Autodesk Inventor part; units mm, degrees
ref_plane "YZ Plane" through (0, 0, 0) normal (1, 0, 0) x (0, 1, 0)
ref_plane "XZ Plane" through (0, 0, 0) normal (0, 1, 0) x (-1, 0, 0)
ref_plane "XY Plane" through (0, 0, 0) normal (0, 0, 1) x (1, 0, 0)
sketch "Sketch1" plane through (0, 0, 0) normal (0, 1, 0) x (-1, 0, 0)
  line L0 (2.2807, -2.5252) -> (-23.1193, -2.5252)
  line L1 (-23.1193, -2.5252) -> (-23.1193, 48.2748)
  line L2 (-23.1193, 48.2748) -> (2.2807, 48.2748)
  line L3 (2.2807, 48.2748) -> (2.2807, -2.5252)
  line L4 (-19.9443, 0.6498) -> (-0.8943, 0.6498)
  line L5 (-0.8943, 0.6498) -> (-0.8943, 45.0998)
  line L6 (-0.8943, 45.0998) -> (-19.9443, 45.0998)
  line L7 (-19.9443, 45.0998) -> (-19.9443, 0.6498)
  point P0 (0, 0)
  dimension "d0" = 25.4
  dimension "d1" = 50.8
  dimension "d2" = 3.175
extrude "Extrusion1" add sketch "Sketch1" along normal blind 762
sketch "Sketch3" plane through (-2.2807, 0, 48.2748) normal (0, 0, 1) x (1, 0, 0)
  line L0 (22.225, 0) -> (3.175, 0) construction
  line L1 (12.7, 0) -> (12.7, 12.7) construction
  line L2 (12.7, 12.7) -> (12.7, 38.1) construction
  line L3 (12.7, 38.1) -> (12.7, 63.5) construction
  circle A0 centre (12.7, 63.5) radius 2.5797
  circle A1 centre (12.7, 38.1) radius 2.5797
  circle A2 centre (12.7, 12.7) radius 2.5797
  line L4 (12.7, 685.8) -> (12.7, 673.1) construction
  circle A3 centre (12.7, 673.1) radius 2.5797
  line L5 (12.7, 673.1) -> (12.7, 647.7) construction
  line L6 (12.7, 647.7) -> (12.7, 622.3) construction
  circle A4 centre (12.7, 647.7) radius 2.5797
  circle A5 centre (12.7, 622.3) radius 2.5797
  point P0 (2.2807, 0)
  dimension "d19" = 12.7
  dimension "d20" = 25.4
  dimension "d21" = 25.4
  dimension "d22" = 5.1594
  dimension "d23" = 5.1594
  dimension "d24" = 5.1594
  dimension "d38" = 12.7
  dimension "d39" = 5.1594
  dimension "d40" = 25.4
  dimension "d41" = 25.4
  dimension "d42" = 5.1594
  dimension "d43" = 5.1594
extrude "Extrusion3" cut sketch "Sketch3" against normal blind 762
sketch "Sketch4" plane through (23.1193, 0, 48.2748) normal (1, 0, 0) x (0, 0, -1)
  line L0 (3.175, 762) -> (47.625, 762) construction
  line L1 (25.4, 762) -> (25.4, 736.6) construction
  point P0 (48.2748, 0)
  dimension "d44" = 25.4
sketch "Sketch5" plane through (-2.2807, 0, -2.5252) normal (-1, 0, 0) x (0, 0, 1)
  circle A0 centre (25.4, 12.7) radius 2.5797
  line L0 (50.8, 0) -> (50.8, 762)
  circle A1 centre (25.4, 38.1) radius 2.5797 construction
  line L1 (50.8, 38.1) -> (38.1, 38.1) construction
  circle A2 centre (25.4, 63.5) radius 2.5797 construction
  line L2 (50.8, 63.5) -> (38.1, 63.5) construction
  circle A3 centre (38.1, 63.5) radius 2.5797
  circle A4 centre (38.1, 38.1) radius 2.5797
  circle A5 centre (38.1, 12.7) radius 2.5797
  line L3 (38.1, 12.7) -> (50.8, 12.7) construction
  circle A6 centre (25.4, 622.3) radius 2.5797 construction
  line L4 (50.8, 622.3) -> (38.1, 622.3) construction
  circle A7 centre (25.4, 647.7) radius 2.5797 construction
  line L5 (50.8, 647.7) -> (38.1, 647.7) construction
  circle A8 centre (25.4, 673.1) radius 2.5797 construction
  line L6 (50.8, 673.1) -> (38.1, 673.1) construction
  circle A9 centre (38.1, 647.7) radius 2.5797
  circle A10 centre (38.1, 622.3) radius 2.5797
  circle A11 centre (38.1, 673.1) radius 2.5797
  point P0 (2.5252, 0)
  dimension "d46" = 12.7
  dimension "d47" = 12.7
  dimension "d48" = 5.1594
  dimension "d49" = 5.1594
  dimension "d50" = 5.1594
  dimension "d51" = 12.7
  dimension "d52" = 12.7
  dimension "d53" = 12.7
  dimension "d54" = 5.1594
  dimension "d55" = 5.1594
  dimension "d56" = 5.1594
extrude "Extrusion4" cut sketch "Sketch5" against normal blind 762 contours A3 | A4 | A5 | A9 | A10 | A11
sketch "Sketch6" plane through (-2.2807, 0, -2.5252) normal (-1, 0, 0) x (0, 0, 1)
  line L0 (47.625, 762) -> (3.175, 762) construction
  line L1 (25.4, 762) -> (25.4, 736.6) construction
  circle A0 centre (25.4, 736.6) radius 14.2875
  point P0 (2.5252, 0)
  dimension "d59" = 25.4
  dimension "d60" = 28.575
extrude "Extrusion5" cut sketch "Sketch6" against normal blind 304.8
sketch "Sketch7" plane through (-2.2807, 0, -2.5252) normal (-1, 0, 0) x (0, 0, 1)
  circle A0 centre (38.1, 12.7) radius 2.5797 construction
  line L0 (38.1, 12.7) -> (38.1, 114.3) construction
  line L1 (38.1, 12.7) -> (38.1, 190.5) construction
  line L2 (38.1, 190.5) -> (12.7, 190.5) construction
  line L3 (38.1, 114.3) -> (12.7, 114.3) construction
  circle A1 centre (38.1, 190.5) radius 2.5797
  circle A2 centre (12.7, 190.5) radius 2.5797
  circle A3 centre (38.1, 114.3) radius 2.5797
  circle A4 centre (12.7, 114.3) radius 2.5797
  point P0 (2.5252, 0)
  dimension "d63" = 101.6
  dimension "d64" = 177.8
  dimension "d65" = 25.4
  dimension "d66" = 25.4
  dimension "d67" = 5.1594
  dimension "d68" = 5.1594
  dimension "d69" = 5.1594
  dimension "d70" = 5.1594
extrude "Extrusion6" cut sketch "Sketch7" against normal blind 50.8
sketch "Sketch8" plane through (-2.2807, 0, -2.5252) normal (-1, 0, 0) x (0, 0, 1)
  line L0 (0, 0) -> (6.5024, 0) construction
  line L1 (47.625, 0) -> (3.175, 0) construction
  line L2 (6.5024, 0) -> (6.5024, 6.5024) construction
  circle A0 centre (6.5024, 6.5024) radius 3.302
  line L3 (6.5024, 6.5024) -> (6.5024, 93.4974) construction
  circle A1 centre (6.5024, 93.4974) radius 3.302
  point P0 (2.5252, 0)
  dimension "d73" = 6.5024
  dimension "d74" = 6.5024
  dimension "d75" = 6.604
  dimension "d76" = 86.995
  dimension "d77" = 6.604
extrude "Extrusion7" cut sketch "Sketch8" against normal blind 50.8
properties part number "30in 1x1 Beam"
Source: CAD feature listing. Evaluate the final solid. Frame: model axes, mm. A direction names the side the tool comes from. Give positions to 0.01 mm unless a question says otherwise; leave off trailing zeros. Write each loop counter-clockwise with the first axis right and the second up, starting at its lowest first coordinate (ties: lowest second). Pieces come first, ordered by that corner, then holes. Notation, with made-up numbers: (33.5, 42.5) - (46.5, 42.5) arc R19 ccw to (46.5, 53.5) - close; hole circle Ø8 at (-12.5, 12). An arc over 180 degrees is marked (long way). One line per item, written item: value. Start each with the question number.
Q1. Section query B-B, the plane z = 22. Return the cut outline in (x, y).
Q2. Set-up query: faces 4 (the face through (19.944, 376, 23)), 5 (the face through (21.51, 722.65, 19.78)). Return all of +Z, -Z, +X, -X, +Y, -Y with unobstructed straight access to the full face (end or side cutting, diameter ignored); none if empty.
Q3. Material intervals for probe 1 along Z at (x, y) = (-1.1, 190.5); probe 2 along Y at (x, z) = (20.5, 3.5); probe 3 along Z at (x, y) = (17.5, 506), sorted ascending. Write a range as from..to.
Q4. Section query C-C, the plane y = 268. Return the cut outline in (x, z), then the cut area to 3 significant figures.
Q5. First-contact query: pin 1 Ø8.5 at (x, y) = (10.42, 63.5) entering from +Z. Flat tip, straight axial feed; report the tip coordinate or a pass-through.
Q6. Section query A-A, the plane y = 736.6. Return the cut outline in (x, z), then the cut area to 3 significant figures.
Q7. Draft query along Z for faces 1 (the face through (0.894, 376, 23)), 2 (the face through (-2.281, 376, 23)), 3 (the face through (10, 376, -2.525)). Return one class per face: +Z half, -Z half, draft (parallel to the pull), parting line (faces both ways), or undercut.
Answer:
1. outline: (-2.28, 0) - (0.89, 0) - (0.89, 722.34) - (-2.28, 722.34) - close; (-2.28, 750.86) - (0.89, 750.86) - (0.89, 762) - (-2.28, 762) - close; (19.94, 0) - (23.12, 0) - (23.12, 722.34) - (19.94, 722.34) - close; (19.94, 750.86) - (23.12, 750.86) - (23.12, 762) - (19.94, 762) - close
2. face 4: +Y, -Y
2. face 5: +X, -X
3. probe 1: z = -2.53..7.6, 12.75..33, 38.15..48.27
3. probe 2: y = 0..3.24, 9.77..90.23, 96.76..762
3. probe 3: z = -2.53..0.65, 45.1..48.27
4. outline: (-2.28, -2.53) - (23.12, -2.53) - (23.12, 48.27) - (-2.28, 48.27) - close; hole (0.89, 0.65) - (19.94, 0.65) - (19.94, 45.1) - (0.89, 45.1) - close
4. area: 444 mm2
5. pin 1: stops at z = 48.27
6. outline: (-2.28, -2.53) - (23.12, -2.53) - (23.12, 8.59) - (19.94, 8.59) - (19.94, 0.65) - (0.89, 0.65) - (0.89, 8.59) - (-2.28, 8.59) - close; (-2.28, 37.16) - (0.89, 37.16) - (0.89, 45.1) - (19.94, 45.1) - (19.94, 37.16) - (23.12, 37.16) - (23.12, 48.27) - (-2.28, 48.27) - close
6. area: 262 mm2
7. face 1: undercut
7. face 2: draft
7. face 3: -Z half
